Could you check a few things on this model? Use its own coordinates, in mm. Face numbers are marked on the shaded views. A direction names the side the tool comes from. Give positions to 0.01 mm unless a question says otherwise; leave off trailing zeros. Order: outer loops, then holes, each group sorted by start corner. A loop starts at its lowest first (then second) coordinate and runs counter-clockwise, first axis right, second up. Notation, with made-up numbers: M -21,17.5 L 20,17.5 A28 cw 20,41.5 Z; hole C -16.75,-22.5 d11. An arc over 180 degrees is marked long. Use a Markdown table: item, result. Add a question column.
Item 1: I'm going to push flat-ended pins straight in: pin 1 Ø6 at (x, y) = (1, 3) entering from -Z; pin 2 Ø7 at (x, y) = (13.5, -6) entering from +Z; pin 3 Ø4.5 at (x, y) = (-12, 6) entering from +Z. Where does each tip first touch, or does it pass through?
Item 2: Suppose I cut it at C-C on y = 0. Write out the boundary of the cut face in (x, z), plus the area to 3 significant figures.
Item 3: Suppose I cut it at A-A on x = 0. Write out the boundary of the cut face in (y, z).
Item 4: If I drill on L1, parallel to Y at x = 13.5, z = 7.5; L2, parallel to Y at x = 13.5, z = 13; L3, parallel to X at y = -6, z = 4.25, over which ranges is the centre line in solid material (lowest first)? Write a range as from..to.
Item 5: Suppose I cut it at D-D on z = 7.5. Write out the boundary of the cut face in (x, y), plus the area to 3 significant figures.
Item 6: If we mould it in two halves opening along Y, with no side actions, what happens to the marked faces 5, 6 and 7? For each: released by +Y, released by -Y, zero draft, split by the parting line, or undercut.
Item 7: For the marked faces 1, 2, 3 and 4, which set-ups out of +Z, -Z, +X, -X, +Y, -Y let a thin tool reach every point of the face, with its end or its side?
Item 8: Suppose I cut it at B-B on z = 5. Write out the boundary of the cut face in (x, y).
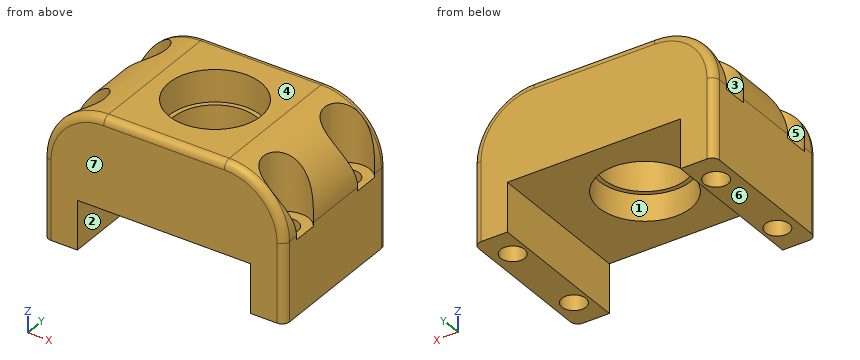
from build123d import *

# Parameters (mm, degrees)
SKETCH3_W           = 32
SKETCH3_H           = 20
SKETCH3_R           = 1.6
BOSS_EXTRUDE1_DEPTH = 18.5
CUT_EXTRUDE1_REACH  = 33.595
SKETCH5_W           = 23
SKETCH5_H           = 6.5
FILLET2_START       = -11
FILLET2_DEPTH       = 22
FILLET1_R           = 1
CUT_EXTRUDE5_REACH  = 38.424
CUT_EXTRUDE5_START  = -10
SKETCH9_R           = 3
SKETCH10_R          = 6.1
CUT_EXTRUDE6_DEPTH  = 4.25
CUT_EXTRUDE7_START  = -3.5
SKETCH12_R          = 6.1
CUT_EXTRUDE7_DEPTH  = 3.5
CUT_EXTRUDE8_REACH  = 23.354
SKETCH13_R          = 5.5


with BuildPart() as part:
    # Sketch3 → Boss-Extrude1 (new body)
    with BuildSketch(Plane.XY):
        Rectangle(SKETCH3_W, SKETCH3_H)
        with Locations((-13.5, 6)):
            Circle(SKETCH3_R, mode=Mode.SUBTRACT)
        with Locations((-13.5, -6)):
            Circle(SKETCH3_R, mode=Mode.SUBTRACT)
        with Locations((13.5, -6)):
            Circle(SKETCH3_R, mode=Mode.SUBTRACT)
        with Locations((13.5, 6)):
            Circle(SKETCH3_R, mode=Mode.SUBTRACT)
    extrude(amount=BOSS_EXTRUDE1_DEPTH)

    # Sketch5 → Cut-Extrude1 (cut, up to next)
    with BuildSketch(Plane(origin=(0, 10, 0), x_dir=(1, 0, 0), z_dir=(0, 1, 0)), mode=Mode.PRIVATE) as cut_extrude1_sk1:
        with Locations((0, -3.25)):
            Rectangle(SKETCH5_W, SKETCH5_H)
    cut_extrude1_tool1 = extrude(cut_extrude1_sk1.sketch, amount=-CUT_EXTRUDE1_REACH, mode=Mode.PRIVATE) & part.part
    add(cut_extrude1_tool1.solids().sort_by_distance((0, 10, 3.25))[0], mode=Mode.SUBTRACT)

    # Fillet2: read off the stored shape, not the designer's step
    # Fillet2 outline → Fillet2 (cut)
    with BuildSketch(Plane(origin=(0, 0, 0), x_dir=(1, 0, 0), z_dir=(0, 1, 0)).offset(FILLET2_START)):
        with BuildLine():
            ThreePointArc((16, -10.5), (13.656854249, -16.156854249), (8, -18.5))
            Line((8, -18.5), (16, -18.5))
            Line((16, -18.5), (16, -10.5))
        make_face()
        with BuildLine():
            Line((-16, -18.5), (-8, -18.5))
            ThreePointArc((-8, -18.5), (-13.656854249, -16.156854249), (-16, -10.5))
            Line((-16, -10.5), (-16, -18.5))
        make_face()
    extrude(amount=FILLET2_DEPTH, mode=Mode.SUBTRACT)

    # Fillet1
    fillet1_edges = [part.edges().sort_by_distance(p)[0] for p in [
        (0, 10, 18.5),
        (0, -10, 18.5),
        (-16, 10, 5.25),
        (16, 10, 5.25),
        (-13.656854249, 10, 16.156854249),
        (13.656854249, 10, 16.156854249),
        (16, -10, 5.25),
        (-16, -10, 5.25),
        (-13.656854249, -10, 16.156854249),
        (13.656854249, -10, 16.156854249),
    ]]
    fillet(fillet1_edges, radius=FILLET1_R)

    # Sketch9 → Cut-Extrude5 (cut, up to next)
    with BuildSketch(Plane(origin=(0, 0, 0), x_dir=(-1, 0, 0), z_dir=(0, 0, -1)).offset(CUT_EXTRUDE5_START), mode=Mode.PRIVATE) as cut_extrude5_sk1:
        with Locations((-13.5, 6)):
            Circle(SKETCH9_R)
    cut_extrude5_tool1 = extrude(cut_extrude5_sk1.sketch, amount=-CUT_EXTRUDE5_REACH, mode=Mode.PRIVATE) & part.part
    # Sketch9 → Cut-Extrude5 (cut, up to next)
    with BuildSketch(Plane(origin=(0, 0, 0), x_dir=(-1, 0, 0), z_dir=(0, 0, -1)).offset(CUT_EXTRUDE5_START), mode=Mode.PRIVATE) as cut_extrude5_sk2:
        with Locations((-13.5, -6)):
            Circle(SKETCH9_R)
    cut_extrude5_tool2 = extrude(cut_extrude5_sk2.sketch, amount=-CUT_EXTRUDE5_REACH, mode=Mode.PRIVATE) & part.part
    # Sketch9 → Cut-Extrude5 (cut, up to next)
    with BuildSketch(Plane(origin=(0, 0, 0), x_dir=(-1, 0, 0), z_dir=(0, 0, -1)).offset(CUT_EXTRUDE5_START), mode=Mode.PRIVATE) as cut_extrude5_sk3:
        with Locations((13.5, -6)):
            Circle(SKETCH9_R)
    cut_extrude5_tool3 = extrude(cut_extrude5_sk3.sketch, amount=-CUT_EXTRUDE5_REACH, mode=Mode.PRIVATE) & part.part
    # Sketch9 → Cut-Extrude5 (cut, up to next)
    with BuildSketch(Plane(origin=(0, 0, 0), x_dir=(-1, 0, 0), z_dir=(0, 0, -1)).offset(CUT_EXTRUDE5_START), mode=Mode.PRIVATE) as cut_extrude5_sk4:
        with Locations((13.5, 6)):
            Circle(SKETCH9_R)
    cut_extrude5_tool4 = extrude(cut_extrude5_sk4.sketch, amount=-CUT_EXTRUDE5_REACH, mode=Mode.PRIVATE) & part.part
    add(cut_extrude5_tool1.solids().sort_by_distance((13.5, 6, 10))[0], mode=Mode.SUBTRACT)
    add(cut_extrude5_tool2.solids().sort_by_distance((13.5, -6, 10))[0], mode=Mode.SUBTRACT)
    add(cut_extrude5_tool3.solids().sort_by_distance((-13.5, -6, 10))[0], mode=Mode.SUBTRACT)
    add(cut_extrude5_tool4.solids().sort_by_distance((-13.5, 6, 10))[0], mode=Mode.SUBTRACT)

    # Sketch10 → Cut-Extrude6 (cut)
    with BuildSketch(Plane.XY.offset(18.5)):
        Circle(SKETCH10_R)
    extrude(amount=-CUT_EXTRUDE6_DEPTH, mode=Mode.SUBTRACT)

    # Sketch12 → Cut-Extrude7 (cut)
    with BuildSketch(Plane(origin=(0, 0, 6.5), x_dir=(-1, 0, 0), z_dir=(0, 0, -1)).offset(CUT_EXTRUDE7_START)):
        with Locations(Location((0, 0, 0), (0, 0, 180))):
            Circle(SKETCH12_R)
    extrude(amount=CUT_EXTRUDE7_DEPTH, mode=Mode.SUBTRACT)

    # Sketch13 → Cut-Extrude8 (cut, up to next)
    with BuildSketch(Plane(origin=(0, 0, 10), x_dir=(-1, 0, 0), z_dir=(0, 0, -1)), mode=Mode.PRIVATE) as cut_extrude8_sk1:
        Circle(SKETCH13_R)
    cut_extrude8_tool1 = extrude(cut_extrude8_sk1.sketch, amount=-CUT_EXTRUDE8_REACH, mode=Mode.PRIVATE) & part.part
    add(cut_extrude8_tool1.solids().sort_by_distance((0, 0, 10))[0], mode=Mode.SUBTRACT)


solid = part.part
Findings below:
| question | item | result |
|---|---|---|
| 1 | pin 1 | stops at z = 6.5 |
| 1 | pin 2 | stops at z = 18.25 |
| 1 | pin 3 | stops at z = 18.31 |
| 2 | outline | M -16,0 L -11.5,0 L -11.5,6.5 L -6.1,6.5 L -6.1,10 L -5.5,10 L -5.5,14.25 L -6.1,14.25 L -6.1,18.5 L -8,18.5 A8 ccw -16,10.5 Z; M 5.5,10 L 6.1,10 L 6.1,6.5 L 11.5,6.5 L 11.5,0 L 16,0 L 16,10.5 A8 ccw 8,18.5 L 6.1,18.5 L 6.1,14.25 L 5.5,14.25 Z |
| 2 | area | 274 mm^2 |
| 3 | outline | M -10,6.5 L -6.1,6.5 L -6.1,10 L -5.5,10 L -5.5,14.25 L -6.1,14.25 L -6.1,18.5 L -9,18.5 A1 ccw -10,17.5 Z; M 5.5,10 L 6.1,10 L 6.1,6.5 L 10,6.5 L 10,17.5 A1 ccw 9,18.5 L 6.1,18.5 L 6.1,14.25 L 5.5,14.25 Z |
| 4 | L1 | y = -10..-7.6, -4.4..4.4, 7.6..10 |
| 4 | L2 | y = -10..-9, -3..3, 9..10 |
| 4 | L3 | x = -16..-15.1, -11.9..-11.5, 11.5..11.9, 15.1..16 |
| 5 | outline | M -16,-9 A1 ccw -15,-10 L 15,-10 A1 ccw 16,-9 L 16,9 A1 ccw 15,10 L -15,10 A1 ccw -16,9 Z; hole C -13.5,-6 d3.2; hole C -13.5,6 d3.2; hole C 0,0 d12.2; hole C 13.5,-6 d3.2; hole C 13.5,6 d3.2 |
| 5 | area | 490 mm^2 |
| 6 | face 5 | undercut |
| 6 | face 6 | zero draft |
| 6 | face 7 | released by -Y |
| 7 | face 1 | -Z |
| 7 | face 2 | -Z, +Y, -Y |
| 7 | face 3 | +Z |
| 7 | face 4 | +Z, +X, -X, +Y, -Y |
| 8 | outline | M -16,-9 A1 ccw -15,-10 L -11.5,-10 L -11.5,10 L -15,10 A1 ccw -16,9 Z; M 11.5,-10 L 15,-10 A1 ccw 16,-9 L 16,9 A1 ccw 15,10 L 11.5,10 Z; hole C -13.5,-6 d3.2; hole C -13.5,6 d3.2; hole C 13.5,-6 d3.2; hole C 13.5,6 d3.2 |
